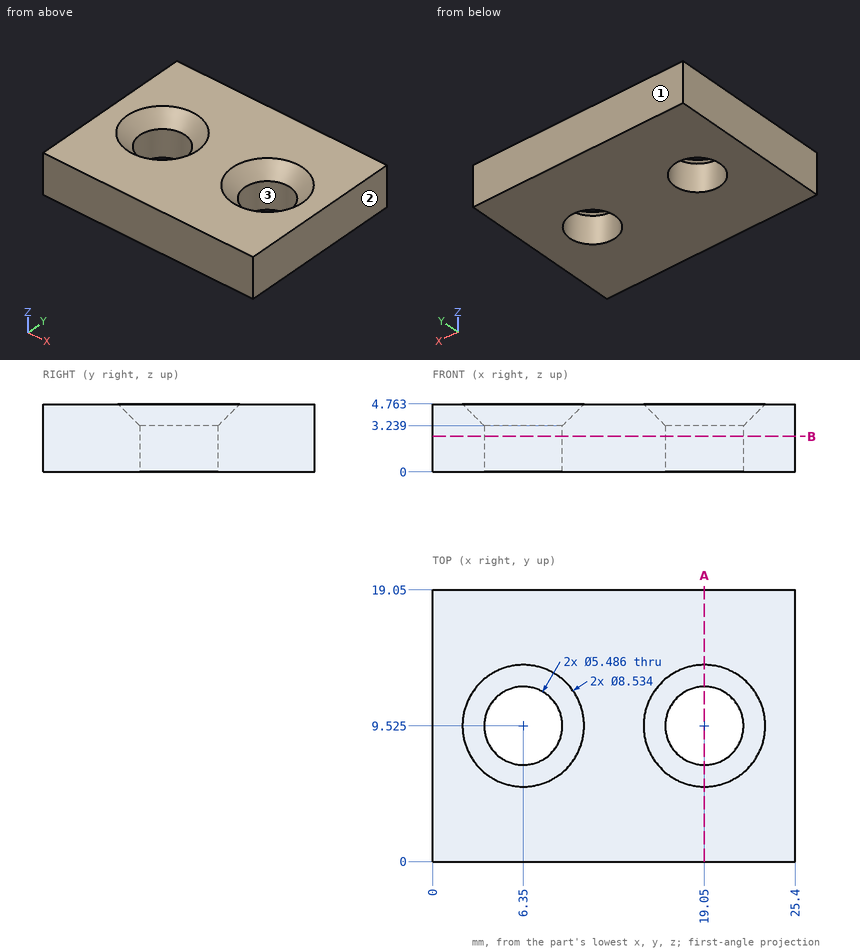
Could you check a few things on this drawing? It's one solid part, dimensions in mm from its lowest x, y, z. Coordinates: 2 decimals unless noted, no trailing zeros. Order: outer loops, then holes, each group sorted by start corner. A loop starts at its lowest first (then second) coordinate and runs counter-clockwise, first axis right, second up. Notation, with made-up numbers: (-20.5, -9.5) - (23.5, -9.5) arc R4 ccw to (23.5, -2.5) - close; hole circle Ø1 at (70, -34). An arc over 180 degrees is marked (long way). Answer as a JSON object with one key per item and string values. Group by question number.
Q1. Will this pin go through, and if not, where does the flat tip stop? P1, Ø9, axis at x = 19.05, y = 9.525, coming from the +Z side.
Q2. Imagine slicing it at A-A (x = 19.05). Please give me the cut outline in (y, z).
Q3. Imagine slicing it at B-B (z = 2.5). Give the number of separate pieces and of enclosed holes in the cut face.
Q4. I need wall thicknesses on line 1 (Y direction, x = 6.35, z = 1.95); line 2 (X direction, y = 10.5, z = 1.8) (1 decimal); line 3 (Y direction, x = 4.5, z = 0.85). Which ranges of each line are inside material? Lowest first, please. Write a range as from..to.
Q5. We'd pull the mould along Y, two halves only. Please class the marked faces 1, 2 and 3: +Y half, -Y half, draft (parallel to the pull), parting line (faces both ways), or undercut.
Determined:
{
 "1": {"P1": "stops at z = 4.76"},
 "2": {"outline": "(0, 0) - (6.78, 0) - (6.78, 3.24) - (5.26, 4.76) - (0, 4.76) - close; (12.27, 0) - (19.05, 0) - (19.05, 4.76) - (13.79, 4.76) - (12.27, 3.24) - close"},
 "3": {"separate pieces": "1", "enclosed holes": "2"},
 "4": {"line 1": "y = 0..6.78, 12.27..19.05", "line 2": "x = 0..3.8, 8.9..16.5, 21.6..25.4", "line 3": "y = 0..7.5, 11.55..19.05"},
 "5": {"face 1": "+Y half", "face 2": "draft", "face 3": "undercut"}
}
